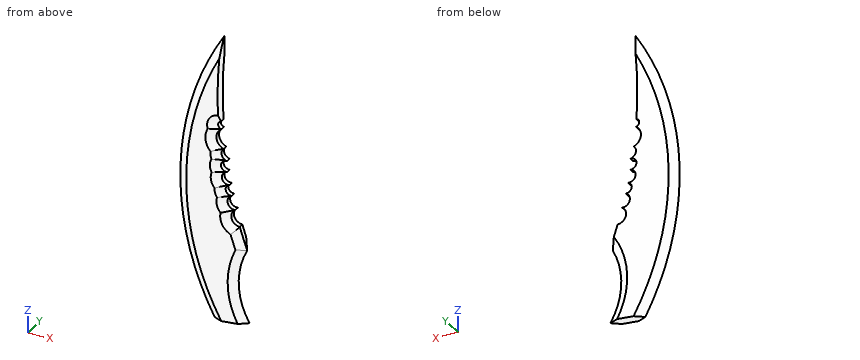
from build123d import *

# Parameters (mm, degrees)
F1_DEPTH    = 1.27
F2_T2_ANGLE = 70.6982594797
F2_T4_ANGLE = 98.1015766654
F2_T6_ANGLE = 98.1015766654
F2_T8_ANGLE = 70.6982594797
F3_SIZE2    = 1.26999
F3_SIZE     = 2.199695


# Not quite as in the source:
# - a fillet or chamfer that OpenCascade refuses, or shapes differently, is made with other operations: its cross-section is extruded or revolved along the edge and cut away or added
# - a fillet or chamfer is up to 0.001 mm smaller than in the source, because OpenCascade refuses the exact size


with BuildPart() as f1:
    # F0 (on Front) → F1 (new body, symmetric)
    with BuildSketch(Plane.XZ):
        with BuildLine():
            ThreePointArc((-24.6599751414, 18.9685343092), (-24.7897166458, 30.8482925644), (-23.6891379404, 42.6776719046))
            ThreePointArc((-23.6891379404, 42.6776719046), (-35.4977812157, 5.0650277845), (-26.6841664691, -33.3599022584))
            Line((-26.6841664691, -33.3599022584), (-16.8598182499, -32.4707999825))
            ThreePointArc((-16.8598182499, -32.4707999825), (-19.7060260634, -23.2610213965), (-17.6819246262, -13.836376369))
            ThreePointArc((-17.6819246262, -13.836376369), (-18.7784432725, -10.7577001108), (-19.7867489636, -7.6490154569))
            ThreePointArc((-19.7867489636, -7.6490154569), (-21.9116415788, -6.0429526618), (-20.9683603212, -3.5520036866))
            ThreePointArc((-20.9683603212, -3.5520036866), (-22.9156863653, -2.1532182096), (-21.8610153861, 0))
            ThreePointArc((-21.8610153861, 0), (-23.4214756824, 1.0408615122), (-22.4479204638, 2.6441765967))
            ThreePointArc((-22.4479204638, 2.6441765967), (-24.4256582154, 3.9784606628), (-23.0913741493, 5.9561984144))
            ThreePointArc((-23.0913741493, 5.9561984144), (-24.6734313076, 7.4086637933), (-23.0913741493, 8.8611291721))
            ThreePointArc((-23.0913741493, 8.8611291721), (-24.4648932463, 10.085402282), (-23.9908037994, 11.8632207636))
            ThreePointArc((-23.9908037994, 11.8632207636), (-25.8325317785, 14.2467515683), (-24.515682055, 16.9558266598))
            ThreePointArc((-24.515682055, 16.9558266598), (-25.3917786695, 17.9045444751), (-24.6599751414, 18.9685343092))
        make_face()
    extrude(amount=F1_DEPTH, both=True)

    # F2: chamfer of 2.54 x 1.4664696837 on 4 edges, made by hand

    # F2_s1 → F2_t2 (revolve, cut)
    with BuildSketch(Plane(origin=(15.8164222993, 0, 20.5345022431), x_dir=(0, 1, 0), z_dir=(0.6102111975, 0, 0.7922387862))):
        Polygon((0.1964696837, 45.0964764528), (-1.27, 42.5564764528), (-1.27, 45.0964764528), align=None)
    revolve(axis=Axis((39.7484673267, -1.27, 2.1011686196), (0, -1, 0)), revolution_arc=F2_T2_ANGLE, mode=Mode.SUBTRACT)

    # F2_s3 → F2_t4 (revolve, cut)
    with BuildSketch(Plane(origin=(10.5087646573, 0, -8.3360437766), x_dir=(0, 1, 0), z_dir=(0.7834430035, 0, -0.6214636436))):
        Polygon((0.1964696837, -37.0387129854), (-1.27, -39.5787129854), (-1.27, -37.0387129854), align=None)
    revolve(axis=Axis((-0.664029112, -1.27, -22.4209338555), (0, 1, 0)), revolution_arc=F2_T4_ANGLE, mode=Mode.SUBTRACT)

    # F2_s5 → F2_t6 (revolve, cut)
    with BuildSketch(Plane(origin=(10.5087646573, 0, -8.3360437766), x_dir=(0, 1, 0), z_dir=(0.7834430035, 0, -0.6214636436))):
        Polygon((-0.1964696837, -37.0387129854), (1.27, -39.5787129854), (1.27, -37.0387129854), align=None)
    revolve(axis=Axis((-0.664029112, 1.27, -22.4209338555), (0, 1, 0)), revolution_arc=F2_T6_ANGLE, mode=Mode.SUBTRACT)

    # F2_s7 → F2_t8 (revolve, cut)
    with BuildSketch(Plane(origin=(15.8164222993, 0, 20.5345022431), x_dir=(0, 1, 0), z_dir=(0.6102111975, 0, 0.7922387862))):
        Polygon((-0.1964696837, 45.0964764528), (1.27, 42.5564764528), (1.27, 45.0964764528), align=None)
    revolve(axis=Axis((39.7484673267, 1.27, 2.1011686196), (0, -1, 0)), revolution_arc=F2_T8_ANGLE, mode=Mode.SUBTRACT)

    # F3 (size 2.1997045256 and 1.27 in the source; OpenCascade refuses exactly that, so slightly less here)
    f3_edges = [f1.edges().sort_by_distance(p)[0] for p in [
        (-25.391779, -1.27, 17.904544),
        (-25.832532, -1.27, 14.246752),
        (-24.464893, -1.27, 10.085402),
        (-24.673431, -1.27, 7.408664),
        (-24.425658, -1.27, 3.978461),
        (-23.421476, -1.27, 1.040862),
        (-22.915686, -1.27, -2.153218),
        (-21.911642, -1.27, -6.042953),
        (-19.304708, -1.27, -9.17292),
    ]]
    f3_side = f1.faces().sort_by_distance((-26.820245, -1.27, -2.285194))[0]
    chamfer(f3_edges, length=F3_SIZE, length2=F3_SIZE2, reference=f3_side)


solid = f1.part
Work out the finished part from the listing and answer in its coordinate system (mm). Give positions to 0.01 mm unless a question says otherwise; leave off trailing zeros. Write each loop counter-clockwise with the first axis right and the second up, starting at its lowest first coordinate (ties: lowest second). Pieces come first, ordered by that corner, then holes.
Q1. The part is cut by section A-A on y = -0.4. Give the vertices of the cut face in (x, z).
Answer:
outline: (-25.68, 16.86) arc R1.73 cw to (-24.7, 19.67) arc R114.63 cw to (-24.03, 40.17) arc R74.27 ccw to (-25.57, -33.26) - (-18, -32.57) arc R20.09 cw to (-18.6, -13.36) arc R115.32 cw to (-20.31, -8.29) arc R2.91 cw to (-22.3, -3.96) arc R2.55 cw to (-23.27, -0.34) arc R2.05 cw to (-23.94, 2.23) arc R2.38 cw to (-24.63, 5.79) arc R2.15 cw to (-24.65, 9.01) arc R2.45 cw to (-25.01, 11.62) arc R3.55 cw to start
Q2. Given pin 1 (3.5 mm diameter, centred on x = -23.22, z = 7.41, fed in from -Y); pin 2 (3 mm diameter, centred on x = -31, z = 25.5, fed in from +Y), each flat-ended and moving along its own axis, determine where each tip first touches the part or whether it passes through.
Answer:
pin 1: stops at y = -0.17
pin 2: stops at y = 1.12
Q3. Straight lines are drawn through the part: L1, parallel to X at y = 0.3, z = 0.5; L2, parallel to X at y = 0.3, z = 9.5; L3, parallel to Z at x = -21.5, y = -0.5. For each, find the intervals that lie inside material, in ascending order.
Answer:
L1: x = -34.68 to -23.17
L2: x = -34.33 to -24.16
L3: z = -32.89 to -7.99
